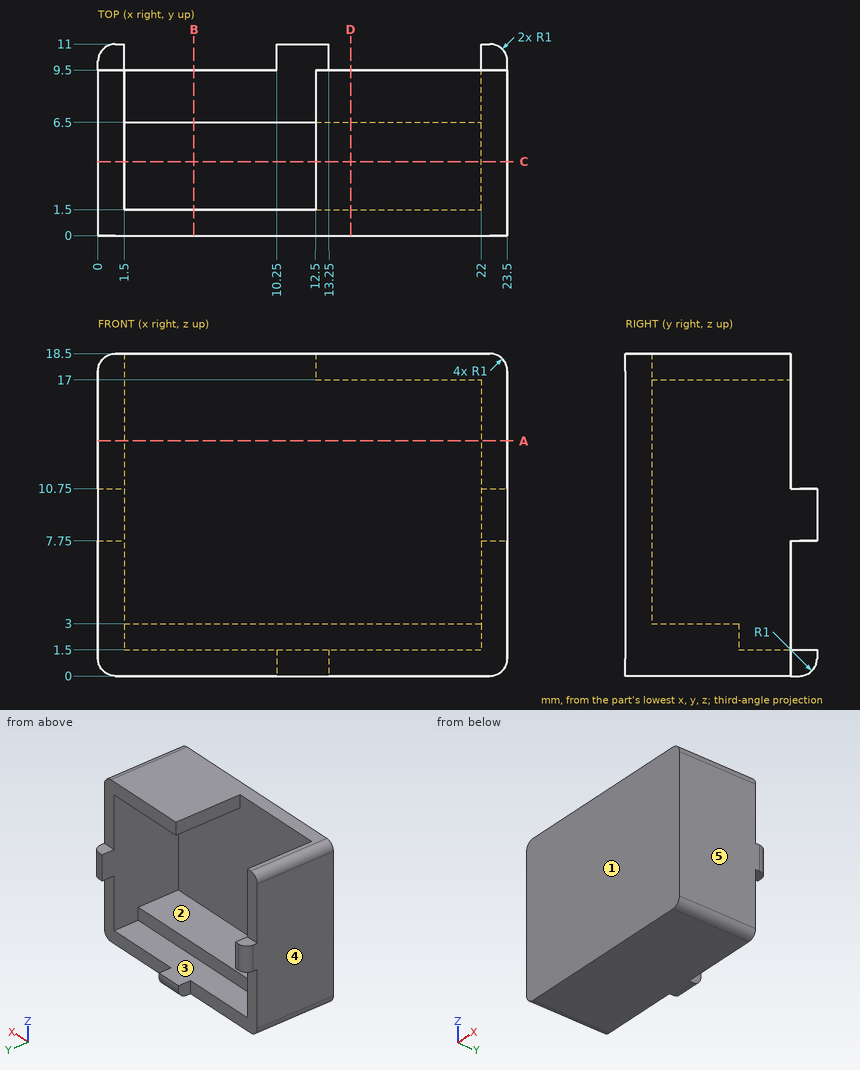
For this review, use the dimensioned drawing (mm, ordinates from the lowest corner) and the shaded views. A direction names the side the tool comes from. Give positions to 0.01 mm unless a question says otherwise; leave off trailing zeros. Loops run counter-clockwise (first coordinate to the right, second up) from the corner with the lowest first, then second, coordinate; pieces in that order, holes last. Notation, with made-up numbers: (75.5, 43.5) -> (95.5, 43.5) arc R17 ccw to (95.5, 70.5) -> close; hole circle Ø7 at (58.5, 41.25). An arc over 180 degrees is marked (long way). One line per question, with ' | ' between items. Start each with the question number.
(1) Insertion check: P1, Ø2.5, axis at x = 15.5, z = 14, coming from the +Y side; P2, Ø2.5, axis at x = 3, z = 3, coming from the +Y side; P3, Ø1.3, axis at x = 7, y = 8.5, coming from the +Z side. Each pin has a flat end and moves straight along its axis. Give the tip position at first contact, or say it passes through.
(2) We need section D-D (x = 14.5). State the section outline as (y, z) points.
(3) We need section C-C (y = 4.25). State the section outline as (x, z) points, and give its area (3 significant figures).
(4) Draft analysis for pull direction X (two halves, no side actions). For the marked faces 3, 4 and 5, state which applies: +X half, -X half, draft (parallel to the pull), parting line (faces both ways), or undercut.
(5) For the marked faces 1 and 2, list the 3-axis set-ups (+Z, -Z, +X, -X, +Y, -Y) from which the entire face can be reached by the end or side of a thin tool; tool diameter is ignored.
(6) We need section B-B (x = 5.5). State the section outline as (y, z) points, and give its area (4 significant figures).
(7) For line 1 (Z direction, x = 16.75, y = 8); line 2 (Z direction, x = 16, y = 5.25); line 3 (X direction, y = 4, z = 6.75), list the stretches that pass through material, from the lowest coordinate up.
(8) We need section A-A (z = 13.5). State the section outline as (x, y) points, and give its area (4 significant figures).
The answers:
1) P1: stops at y = 1.5 | P2: stops at y = 6.5 | P3: stops at z = 1.5
2) outline: (0, 0) -> (9.5, 0) -> (9.5, 1.5) -> (6.5, 1.5) -> (6.5, 3) -> (1.5, 3) -> (1.5, 17) -> (9.5, 17) -> (9.5, 18.5) -> (0, 18.5) -> close
3) outline: (0, 1) arc R1 ccw to (1, 0) -> (22.5, 0) arc R1 ccw to (23.5, 1) -> (23.5, 17.5) arc R1 ccw to (22.5, 18.5) -> (12.5, 18.5) -> (12.5, 17) -> (22, 17) -> (22, 3) -> (1.5, 3) -> (1.5, 18.5) -> (1, 18.5) arc R1 ccw to (0, 17.5) -> close | area: 130 mm^2
4) face 3: undercut | face 4: -X half | face 5: +X half
5) face 1: +Z, -Z, +X, -X, -Y | face 2: +Y
6) outline: (0, 0) -> (9.5, 0) -> (9.5, 1.5) -> (6.5, 1.5) -> (6.5, 3) -> (1.5, 3) -> (1.5, 18.5) -> (0, 18.5) -> close | area: 47.25 mm^2
7) line 1: z = 0 to 1.5, 17 to 18.5 | line 2: z = 0 to 3, 17 to 18.5 | line 3: x = 0 to 1.5, 22 to 23.5
8) outline: (0, 0) -> (23.5, 0) -> (23.5, 9.5) -> (22, 9.5) -> (22, 1.5) -> (1.5, 1.5) -> (1.5, 9.5) -> (0, 9.5) -> close | area: 59.25 mm^2
